Could you check a few things on this model? Use its own coordinates, in mm. A direction names the side the tool comes from. Give positions to 0.01 mm unless a question says otherwise; leave off trailing zeros. Write each loop counter-clockwise with the first axis right and the second up, starting at its lowest first coordinate (ties: lowest second). Pieces come first, ordered by that corner, then holes. Notation, with made-up numbers: (49.5, 24.25) -> (79.5, 24.25) arc R28 ccw to (79.5, 60.25) -> close; hole circle Ø9 at (43.5, 59). An arc over 180 degrees is marked (long way). Write item = value, one per line. Start each with the question number.
Autodesk Inventor part; units mm, degrees
ref_plane "YZ Plane" through (0, 0, 0) normal (1, 0, 0) x (0, 1, 0)
ref_plane "XZ Plane" through (0, 0, 0) normal (0, 1, 0) x (-1, 0, 0)
ref_plane "XY Plane" through (0, 0, 0) normal (0, 0, 1) x (1, 0, 0)
sketch "Sketch1" plane through (0, 0, 0) normal (0, 0, 1) x (1, 0, 0)
  line L0 (-6.35, 5) -> (6.35, 5)
  line L1 (6.35, 5) -> (6.35, -5)
  line L2 (6.35, -5) -> (-6.35, -5)
  line L3 (-6.35, -5) -> (-6.35, 5)
  line L4 (-6.35, 5) -> (6.35, -5) construction
  line L5 (6.35, 5) -> (-6.35, -5) construction
  line L6 (-2.4214, 4.3746) -> (-6.35, 2.2)
  line L7 (-2.4214, -4.3746) -> (-6.35, -2.2)
  line L8 (0, -5) -> (0, 5)
  line L9 (2.4214, 4.3746) -> (6.35, 2.2)
  line L10 (2.4214, -4.3746) -> (6.35, -2.2)
  line L11 (-6.35, 2.2) -> (-6.35, -2.2)
  line L12 (6.35, -2.2) -> (6.35, 2.2)
  arc A0 (-2.4214, -4.3746) -> (2.4214, -4.3746) centre (0, 0) ccw
  arc A1 (2.4214, 4.3746) -> (-2.4214, 4.3746) centre (0, 0) ccw
  point P0 (-1.2915, 5)
  point P1 (-1.2915, -5)
  point P2 (1.2915, 5)
  point P3 (1.2915, -5)
  dimension "d0" = 12.7
  dimension "d1" = 10
  dimension "d3" = 2.8
  dimension "d4" = 2.8
extrude "Extrusion1" add sketch "Sketch1" along normal blind 1.2 contours A1 L9 L1 L10 A0 L8 | L8 A0 L7 L3 L6 A1
sketch "Sketch2" plane through (0, 0, 1.2) normal (0, 0, 1) x (1, 0, 0)
  arc A0 (2.4214, 4.3746) -> (-2.4214, 4.3746) centre (0, 0) ccw
  circle A1 centre (0, 0) radius 3.5
  circle A2 centre (0, 0) radius 4.5
  dimension "d7" = 7
  dimension "d8" = 1
extrude "Extrusion2" add sketch "Sketch2" along normal blind 0.5 contours A1 | A2
sketch "Sketch3" plane through (0, 0, 1.7) normal (0, 0, 1) x (1, 0, 0)
  circle A0 centre (0, 0) radius 4.5
  circle A1 centre (0, 0) radius 3.5
  dimension "d11" = 7
extrude "Extrusion3" add sketch "Sketch3" along normal blind 2.5 contours A1
sketch "Sketch4" plane through (0, 0, 4.2) normal (0, 0, 1) x (1, 0, 0)
  circle A0 centre (0, 0) radius 4.5
  dimension "d14" = 9
extrude "Extrusion4" add sketch "Sketch4" along normal blind 0.8
fillet "Fillet1" radius 0.5 1 edges at (-4.5, 0, 1.7)
sketch "Sketch5" plane through (0, 0, 1.2) normal (0, 0, 1) x (1, 0, 0)
  circle A0 centre (0, 0) radius 4.5
  line L0 (-6.35, 2.2) -> (-6.35, -2.2)
  line L1 (-6.35, -2.2) -> (-2.4214, -4.3746)
  arc A1 (-2.4214, -4.3746) -> (2.4214, -4.3746) centre (0, 0) ccw
  line L2 (2.4214, -4.3746) -> (6.35, -2.2)
  line L3 (6.35, -2.2) -> (6.35, 2.2)
  line L4 (6.35, 2.2) -> (2.4214, 4.3746)
  arc A2 (2.4214, 4.3746) -> (-2.4214, 4.3746) centre (0, 0) ccw
  line L5 (-2.4214, 4.3746) -> (-6.35, 2.2)
  line L6 (-6.35, 2.2) -> (-6.35, -2.2)
  line L7 (-6.35, 1) -> (-6.15, 1)
  line L8 (-6.15, 1) -> (-6.15, -1)
  line L9 (-6.15, -1) -> (-6.35, -1)
  line L10 (-6.35, -1) -> (-6.35, 1)
  line L11 (6.35, -1) -> (6.15, -1)
  line L12 (6.15, -1) -> (6.15, 1)
  line L13 (6.15, 1) -> (6.35, 1)
  line L14 (6.35, 1) -> (6.35, -1)
  point P0 (6.35, 0)
  point P1 (-6.35, 0)
  dimension "d18" = 2
  dimension "d19" = 2
  dimension "d20" = 0.2
  dimension "d21" = 0.2
extrude "Extrusion5" cut sketch "Sketch5" against normal through all contours L7 L8 L9 L0 | L3 L11 L12 L13
sketch "Sketch6" plane through (0, 0, 1.2) normal (0, 0, 1) x (1, 0, 0)
  line L0 (-6.15, -1) -> (-6.35, -1)
  line L1 (-6.35, -1) -> (-6.35, -2.2)
  line L2 (-6.35, -2.2) -> (-2.4214, -4.3746)
  arc A0 (-2.4214, -4.3746) -> (2.4214, -4.3746) centre (0, 0) ccw
  line L3 (2.4214, -4.3746) -> (6.35, -2.2)
  line L4 (6.35, -2.2) -> (6.35, -1)
  line L5 (6.35, -1) -> (6.15, -1)
  line L6 (6.15, -1) -> (6.15, 1)
  line L7 (6.15, 1) -> (6.35, 1)
  line L8 (6.35, 1) -> (6.35, 2.2)
  line L9 (6.35, 2.2) -> (2.4214, 4.3746)
  arc A1 (2.4214, 4.3746) -> (-2.4214, 4.3746) centre (0, 0) ccw
  line L10 (-2.4214, 4.3746) -> (-6.35, 2.2)
  line L11 (-6.35, 2.2) -> (-6.35, 1)
  line L12 (-6.35, 1) -> (-6.15, 1)
  line L13 (-6.15, 1) -> (-6.15, -1)
  circle A2 centre (0, 0) radius 4.5
  line L14 (-6.15, 1) -> (-4.65, 1)
  line L15 (-4.65, 1) -> (-4.65, -1)
  line L16 (-4.65, -1) -> (-6.15, -1)
  line L17 (-6.15, -1) -> (-6.15, 1)
  line L18 (6.15, -1) -> (4.65, -1)
  line L19 (4.65, -1) -> (4.65, 1)
  line L20 (4.65, 1) -> (6.15, 1)
  line L21 (6.15, 1) -> (6.15, -1)
  dimension "d24" = 1.5
  dimension "d25" = 1.5
extrude "Extrusion6" cut sketch "Sketch6" against normal blind 0.2 contours L13 L14 L15 L16 | L18 L19 L20 L6
sketch "Sketch7" plane through (0, 0, 0) normal (0, 0, -1) x (-1, 0, 0)
  circle A0 centre (0, 0) radius 4
  line L0 (6.35, -1) -> (6.15, -1)
  line L1 (6.15, -1) -> (6.15, 1)
  line L2 (6.15, 1) -> (6.35, 1)
  line L3 (6.35, 2.2) -> (6.35, 1)
  line L4 (2.4214, 4.3746) -> (6.35, 2.2)
  arc A1 (2.4214, 4.3746) -> (-2.4214, 4.3746) centre (0, 0) ccw
  line L5 (-6.35, 2.2) -> (-2.4214, 4.3746)
  line L6 (-6.35, 1) -> (-6.35, 2.2)
  line L7 (-6.35, 1) -> (-6.15, 1)
  line L8 (-6.15, 1) -> (-6.15, -1)
  line L9 (-6.15, -1) -> (-6.35, -1)
  line L10 (-6.35, -2.2) -> (-6.35, -1)
  line L11 (-2.4214, -4.3746) -> (-6.35, -2.2)
  arc A2 (-2.4214, -4.3746) -> (2.4214, -4.3746) centre (0, 0) ccw
  line L12 (6.35, -2.2) -> (2.4214, -4.3746)
  line L13 (6.35, -1) -> (6.35, -2.2)
  line L14 (6.15, -1) -> (4.65, -1)
  line L15 (4.65, -1) -> (4.65, 1)
  line L16 (4.65, 1) -> (6.15, 1)
  line L17 (6.15, 1) -> (6.15, -1)
  line L18 (-6.15, 1) -> (-4.65, 1)
  line L19 (-4.65, 1) -> (-4.65, -1)
  line L20 (-4.65, -1) -> (-6.15, -1)
  line L21 (-6.15, -1) -> (-6.15, 1)
  dimension "d28" = 1.5
  dimension "d29" = 1.5
extrude "Extrusion7" cut sketch "Sketch7" against normal blind 0.1 contours L14 L15 L16 L1 | L8 L18 L19 L20
properties part number "SDR1005"
(1) On a 3-axis mill with a long thin cutter (end or side, diameter ignored), from which of +Z, -Z, +X, -X, +Y, -Y can I reach the whole of each face in a straight line? I mean faces 1 (the cylindrical face through (-0.59, -4.46, 4.59)), 2 (the flat face through (-5, 0, 0.1)), 3 (the flat face through (6.15, 0, 0.6)), 4 (the cylindrical face through (3.233, 1.341, 2.932)), 5 (the flat face through (5, 0, 0.1)). Say none if no direction works.
(2) We'd pull the mould along Y, two halves only. Please class faces 6 (the flat face through (0, -4, 4.2)), 7 (the flat face through (-4.36, -3.3, 0.59)), 8 (the flat face through (5, 0, 1)), 9 (the flat face through (-4.36, 3.3, 0.59)): released by +Y, released by -Y, zero draft, split by the parting line, or undercut.
(3) Imagine slicing it at D-D (x = -5). Please give me the cut outline in (y, z), then the cut area to 3 significant figures.
(4) I'm going to push flat-ended pins straight in: pin 1 (1.3 mm diameter, centred on x = 6, z = 0.5, fed in from +Y); pin 2 (1.2 mm diameter, centred on x = 6, y = 0, fed in from +Z); pin 3 (1.3 mm diameter, centred on x = -5.5, z = 1, fed in from -Y). Where does each tip first touch, or does it pass through?
(5) Imagine slicing it at C-C (z = 2.2). Please give me the cut outline in (x, y), then the cut area to 3 significant figures.
(6) If I drill on line 1 along Z through (x, y) = (-3, -3.5); line 2 along Z through (x, y) = (-2.5, -3.5); line 3 along X through (y, z) = (-1.75, 4.7), over which ranges is the centre line in solid material (lowest first)? Write a range as from..to.
Answers below:
q1.face_1 = +Z
q1.face_2 = -Z, -X
q1.face_3 = +Z, -Z, +X
q1.face_4 = none
q1.face_5 = -Z, +X
q2.face_6 = zero draft
q2.face_7 = released by -Y
q2.face_8 = undercut
q2.face_9 = released by +Y
q3.outline = (-2.95, 0) -> (-1, 0) -> (-1, 0.1) -> (1, 0.1) -> (1, 0) -> (2.95, 0) -> (2.95, 1.2) -> (1, 1.2) -> (1, 1) -> (-1, 1) -> (-1, 1.2) -> (-2.95, 1.2) -> close
q3.area = 6.47 mm^2
q4.pin_1 = 2.75
q4.pin_2 = 1
q4.pin_3 = -3.03
q5.outline = circle Ø7 at (0, 0)
q5.area = 38.5 mm^2
q6.line_1 = 0..1.2
q6.line_2 = 0..1.6, 4.2..5
q6.line_3 = -4.15..4.15
